```python
from build123d import *

# Parameters (mm, degrees)
F1_DEPTH = 8
F3_D     = 4
F3_DEPTH = 5
F3_TIP   = 1.2017212381
F4_SIZE  = 1
F5_R     = 5


with BuildPart() as f1:
    # F0 (on Top) → F1 (new body)
    with BuildSketch(Plane.XY):
        with BuildLine():
            Line((3.1, 3.1), (40.8826369013, 3.1))
            ThreePointArc((40.8826369013, 3.1), (28.9913780286, 28.9913780286), (3.1, 40.8826369013))
            Line((3.1, 40.8826369013), (3.1, 3.1))
        make_face()
    extrude(amount=F1_DEPTH)

    # F3
    with Locations(Plane.XY.offset(8)):
        with Locations((14, 14), (24, 24)):
            Hole(F3_D / 2, depth=F3_DEPTH)
            with Locations((0, 0, -(F3_DEPTH + F3_TIP / 2))):  # 118° drill point
                Cone(0, F3_D / 2, F3_TIP, mode=Mode.SUBTRACT)

    # F4
    f4_edges = [f1.edges().sort_by_distance(p)[0] for p in [
        (3.1, 3.1, 4),
        (21.991318, 3.1, 8),
        (3.1, 21.991318, 8),
    ]]
    chamfer(f4_edges, length=F4_SIZE)

    # F5
    f5_edges = [f1.edges().sort_by_distance(p)[0] for p in [
        (28.991378, 28.991378, 0),
    ]]
    fillet(f5_edges, radius=F5_R)


solid = f1.part
```
For this review, take the finished solid that the model builds, in its own axes (mm). A direction names the side the tool comes from. Round coordinates to 2 decimals unless told otherwise and drop trailing zeros. Loops run counter-clockwise (first coordinate to the right, second up) from the corner with the lowest first, then second, coordinate; pieces in that order, holes last.
(1) We need section B-B (z = 0.5). Give the boundary of the cut face in (x, y).
Returned:
outline: (3.1, 4.1) - (4.1, 3.1) - (38.05, 3.1) arc R38.18 ccw to (3.1, 38.05) - close
(2) Mouldability with a two-part tool opening along X and no side actions: class faces 1 (the cylindrical face through (25.6, 22.8, 5.5)), 2 (the flat face through (16, 16, 0)), 3 (the cylindrical face through (29.28, 28.7, 6.48)) as released by +X, released by -X, zero draft, split by the parting line, or undercut.
Returned:
face 1: undercut
face 2: zero draft
face 3: released by +X
(3) Tool access review of faces 4 (the cylindrical face through (14, 16, 5)), 5 (the flat face through (3.8, 3.8, 7.4)): name each direction out of +Z, -Z, +X, -X, +Y, -Y from which nothing blocks a thin tool from reaching the whole face with its end or side.
Returned:
face 4: +Z
face 5: +Z, -X, -Y
(4) Clearance check with a flat-ended pin moving along its axis: P1, Ø2.5, axis at x = 24, y = 24, coming from the +Z side. State where the tip first meets the part, or that it passes through.
Returned:
P1: stops at z = 2.55
(5) Wall thickness on line 1 along X through (y, z) = (24, 4.45); line 2 along Y through (x, z) = (24, 4.25); line 3 along Y through (x, z) = (14, 5.95): over which ranges is each line inside the solid? List them lowest first.
Returned:
line 1: x = 3.1 to 22, 26 to 33.2
line 2: y = 3.1 to 22, 26 to 33.17
line 3: y = 3.1 to 12, 16 to 38.54
(6) We need section A-A (z = 3.5). Give the boundary of the cut face in (x, y), plus the area to 3 significant figures.
Returned:
outline: (3.1, 4.1) - (4.1, 3.1) - (40.65, 3.1) arc R40.77 ccw to (3.1, 40.65) - close; hole circle Ø4 at (14, 14); hole circle Ø4 at (24, 24)
area: 1,040 mm2
